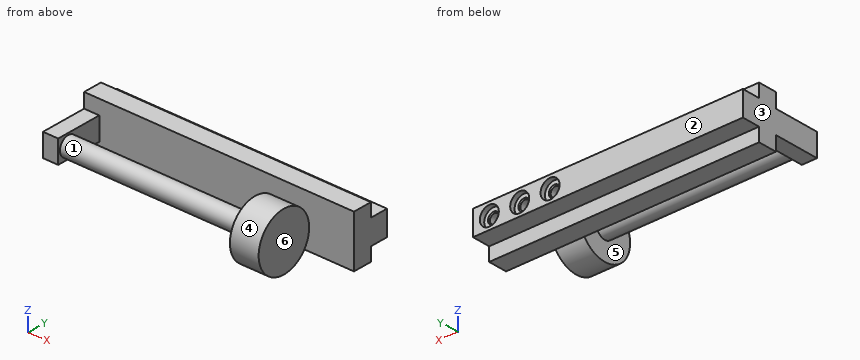
Autodesk Inventor part; units mm, degrees
ref_plane "ANBAU_XY" through (23.25, -9.2, 0) normal (1, 0, 0) x (0, 0, -1)
ref_plane "ANBAU_YZ" through (23.25, -9.2, 0) normal (0, 0, -1) x (0, 1, 0)
ref_plane "ANBAU_ZX" through (23.25, -9.2, 0) normal (0, 1, 0) x (1, 0, 0)
sketch "Skizze_1" plane through (-37.55, 0, 0) normal (1, 0, 0) x (0, 0, -1)
  line L0 (-6.8, 5) -> (-6.8, 0)
  line L1 (-6.8, 0) -> (6.8, 0)
  line L2 (6.8, 0) -> (6.8, 5)
  line L3 (6.8, 5) -> (3.25, 5)
  line L4 (3.25, 5) -> (3.25, 9.8)
  line L5 (3.25, 9.8) -> (-3.25, 9.8)
  line L6 (-3.25, 9.8) -> (-3.25, 5)
  line L7 (-3.25, 5) -> (-6.8, 5)
extrude "Extrusion1" add sketch "Skizze_1" along normal blind 71.1
sketch "Skizze_2" plane through (0, 0, 0) normal (0, 0, 1) x (1, 0, 0)
  line L0 (-37.55, 7) -> (-37.55, -12.2)
  line L1 (-37.55, -12.2) -> (-33.55, -12.2)
  line L2 (-33.55, -12.2) -> (-33.55, 7)
  line L3 (-33.55, 7) -> (-37.55, 7)
extrude "Extrusion2" add sketch "Skizze_2" along normal mid plane 6
sketch "Sketch_1" plane through (0, 0, 0) normal (0, 0, 1) x (1, 0, 0)
  line L0 (23.25, -9.2) -> (-33.55, -9.2)
  line L1 (-33.55, -9.2) -> (-33.55, -6.7)
  line L2 (-33.55, -6.7) -> (15.6767, -6.7)
  line L3 (15.6767, -6.7) -> (15.6767, -1.7)
  line L4 (15.6767, -1.7) -> (23.25, -1.7)
  line L5 (23.25, -1.7) -> (23.25, -9.2)
  line L6 (23.25, -9.2) -> (-33.55, -9.2)
revolve "Revolution1" add sketch "Sketch_1" angle 360 about axis through (23.25, -9.2, 0) along (1, 0, 0)
sketch "Sketch_3" plane through (29.25, 0, 0) normal (1, 0, 0) x (0, 0, -1)
  line L0 (0, 9.8) -> (0, 0.6401)
  line L1 (0, 0.6401) -> (-1.2295, 1.35)
  line L2 (-1.2295, 1.35) -> (-1.2295, 8.2295)
  line L3 (-1.2295, 8.2295) -> (-1.5, 8.5)
  line L4 (-1.5, 8.5) -> (-2.5, 8.5)
  line L5 (-2.5, 8.5) -> (-2.5, 9.8)
  line L6 (-2.5, 9.8) -> (0, 9.8)
  line L7 (0, 9.8) -> (0, 0.6401)
revolve "Revolution2" cut sketch "Sketch_3" angle 360 about axis through (29.25, 9.8, 0) along (0, 1, 0)
thread "Thread1"
pattern_linear "Rectangular Pattern1" count 3 spacing 8 along (-1, 0, 0) of "Revolution2"
ref_plane "ANBAU_XY" through (23.25, -9.2, 0) normal (1, 0, 0) x (0, 0, -1)
ref_plane "ANBAU_YZ" through (23.25, -9.2, 0) normal (0, 0, -1) x (0, 1, 0)
ref_plane "ANBAU_ZX" through (23.25, -9.2, 0) normal (0, 1, 0) x (1, 0, 0)
ref_plane "SCHRAUBE_1_XY" through (29.25, 8.5, 0) normal (0, 1, 0) x (1, 0, 0)
ref_plane "SCHRAUBE_1_YZ" through (29.25, 8.5, 0) normal (1, 0, 0) x (0, 0, -1)
ref_plane "SCHRAUBE_1_ZX" through (29.25, 8.5, 0) normal (0, 0, -1) x (0, 1, 0)
ref_plane "SCHRAUBE_2_XY" through (21.25, 8.5, 0) normal (0, 1, 0) x (1, 0, 0)
ref_plane "SCHRAUBE_2_YZ" through (21.25, 8.5, 0) normal (1, 0, 0) x (0, 0, -1)
ref_plane "SCHRAUBE_2_ZX" through (21.25, 8.5, 0) normal (0, 0, -1) x (0, 1, 0)
ref_plane "SCHRAUBE_3_XY" through (13.25, 8.5, 0) normal (0, 1, 0) x (1, 0, 0)
ref_plane "SCHRAUBE_3_YZ" through (13.25, 8.5, 0) normal (1, 0, 0) x (0, 0, -1)
ref_plane "SCHRAUBE_3_ZX" through (13.25, 8.5, 0) normal (0, 0, -1) x (0, 1, 0)
ref_plane "ZBHJAW1_XY" through (29.25, 8.5, 0) normal (0, -1, 0) x (1, 0, 0)
ref_plane "ZBHJAW1_YZ" through (29.25, 8.5, 0) normal (1, 0, 0) x (0, 0, 1)
ref_plane "ZBHJAW1_ZX" through (29.25, 8.5, 0) normal (0, 0, 1) x (0, -1, 0)
ref_plane "ZBHJAW2_XY" through (13.25, 8.5, 0) normal (0, -1, 0) x (1, 0, 0)
ref_plane "ZBHJAW2_YZ" through (13.25, 8.5, 0) normal (1, 0, 0) x (0, 0, 1)
ref_plane "ZBHJAW2_ZX" through (13.25, 8.5, 0) normal (0, 0, 1) x (0, -1, 0)
properties part number "3385160 HGPL-BAC-14-40---(J)"
Build history of the part. All positions in model axes, mm. Face numbers are marked on the shaded views. A direction names the side the tool comes from. Coordinates: 2 decimals unless noted, no trailing zeros. Write each loop counter-clockwise with the first axis right and the second up, starting at its lowest first coordinate (ties: lowest second). Pieces come first, ordered by that corner, then holes.
(1) Mould opens along Y. For the marked faces 1, 2 and 3 say: pulls with the +Y half, pulls with the -Y half, needs draft (parallel to the pull), parting line crosses it, or undercut.
(2) Cut at D-D on x = 25.5. List the corners of the cut face in (y, z).
(3) Cut at B-B on y = -9.2. List the corners of the cut face in (x, z), and give its area (3 significant figures).
(4) Cut at C-C on y = -4. List the corners of the cut face in (x, z), and give its area (3 significant figures).
(5) Cut at A-A on x = -32. List the corners of the cut face in (y, z).
(6) 3-axis set-ups, long thin cutter, end or side, ignore diameter. For the marked faces 4, 5 and 6: which of +Z, -Z, +X, -X, +Y, -Y reach the whole face in a straight line?
(7) Drill centre lines: line 1 (X direction, y = 9.45, z = 0); line 2 (X direction, y = 3.25, z = 0); line 3 (X direction, y = -4, z = 0). Where is each one in solid material? Low to high.
(8) Pin check, flat tips, straight feed: pin 1 Ø1.5 at (x, z) = (22.5, -1) entering from +Y; pin 2 Ø1.1 at (x, z) = (-17.5, 6) entering from +Y; pin 3 Ø1.5 at (x, z) = (13.25, 0) entering from -Y. Stop position of each tip, or through.
Working result:
1. face 1: undercut
1. face 2: pulls with the +Y half
1. face 3: needs draft
2. outline: (0, -6.8) - (5, -6.8) - (5, -3.25) - (9.8, -3.25) - (9.8, 3.25) - (5, 3.25) - (5, 6.8) - (0, 6.8) - close
3. outline: (-37.55, -3) - (-33.55, -3) - (-33.55, -2.5) - (15.68, -2.5) - (15.68, -7.5) - (23.25, -7.5) - (23.25, 7.5) - (15.68, 7.5) - (15.68, 2.5) - (-33.55, 2.5) - (-33.55, 3) - (-37.55, 3) - close
3. area: 384 mm2
4. outline: (-37.55, -3) - (-33.55, -3) - (-33.55, 3) - (-37.55, 3) - close; (15.68, -5.4) - (23.25, -5.4) - (23.25, 5.4) - (15.68, 5.4) - close
4. area: 106 mm2
5. outline: circle Ø5 at (-9.2, 0); (0, -6.8) - (5, -6.8) - (5, -3.25) - (9.8, -3.25) - (9.8, 3.25) - (5, 3.25) - (5, 6.8) - (0, 6.8) - close
6. face 4: +X
6. face 5: none
6. face 6: +Z, -Z, +X, -Y
7. line 1: x = -37.55 to 10.75, 15.75 to 18.75, 23.75 to 26.75, 31.75 to 33.55
7. line 2: x = -37.55 to 12.02, 14.48 to 20.02, 22.48 to 28.02, 30.48 to 33.55
7. line 3: x = -37.55 to -33.55, 15.68 to 23.25
8. pin 1: stops at y = 8.5
8. pin 2: stops at y = 5
8. pin 3: stops at y = -11.7
